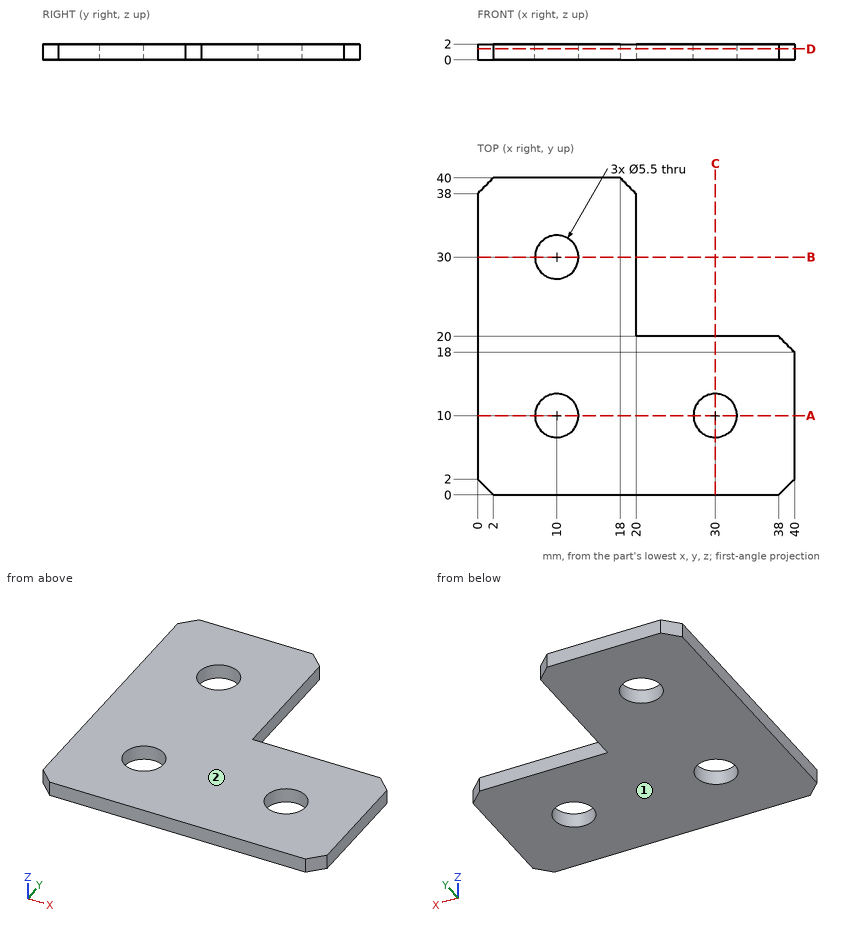
Study the drawing (mm; zero at the part's minimum x, y, z) and answer. Give positions to 0.01 mm unless a question says otherwise; leave off trailing zeros. Write each loop counter-clockwise with the first axis right and the second up, starting at its lowest first coordinate (ties: lowest second). Pieces come first, ordered by that corner, then holes. Notation, with made-up numbers: (59.25, 74.5) - (92.25, 74.5) arc R27 ccw to (92.25, 101.5) - close; hole circle Ø8 at (59.5, -34.75). An arc over 180 degrees is marked (long way). Use CSV: the item, a comma, the result in double quotes. Start each with the question number.
(1) Consider line 1 along Y through (x, z) = (10, 0.85); line 2 along Y through (x, z) = (30, 0.95). Determine where each line is inside the solid, lowest interval first.
(2) Given P1, Ø6.5, axis at x = 30, y = 10, coming from the +Z side, flat-ended and moving along its own axis, determine where the tip first touches the part or whether it passes through.
(3) Find section A-A (y = 10). Give the vertices of the cut face in (x, z).
(4) Find section B-B (y = 30). Give the vertices of the cut face in (x, z), plus the area to 3 significant figures.
(5) Determine the mould class of the marked faces 1 and 2 for opening direction Z: +Z half, -Z half, draft (parallel to the pull), parting line (faces both ways), or undercut.
(6) Find section D-D (z = 1.4). Give the vertices of the cut face in (x, y).
Findings below:
1,line 1,"0 to 7.25, 12.75 to 27.25, 32.75 to 40"
1,line 2,"0 to 7.25, 12.75 to 20"
2,P1,"z = 2"
3,outline,"(0, 0) - (7.25, 0) - (7.25, 2) - (0, 2) - close; (12.75, 0) - (27.25, 0) - (27.25, 2) - (12.75, 2) - close; (32.75, 0) - (40, 0) - (40, 2) - (32.75, 2) - close"
4,outline,"(0, 0) - (7.25, 0) - (7.25, 2) - (0, 2) - close; (12.75, 0) - (20, 0) - (20, 2) - (12.75, 2) - close"
4,area,"29.0 mm2"
5,face 1,"-Z half"
5,face 2,"+Z half"
6,outline,"(0, 2) - (2, 0) - (38, 0) - (40, 2) - (40, 18) - (38, 20) - (20, 20) - (20, 38) - (18, 40) - (2, 40) - (0, 38) - close; hole circle Ø5.5 at (10, 10); hole circle Ø5.5 at (10, 30); hole circle Ø5.5 at (30, 10)"
